CAD build for the part. Positions are in the model's coordinates, mm. A direction names the side the tool comes from. Give positions to 0.01 mm unless a question says otherwise; leave off trailing zeros. Order: outer loops, then holes, each group sorted by start corner. A loop starts at its lowest first (then second) coordinate and runs counter-clockwise, first axis right, second up.
Item 1: Flat gauge pins, fed straight in: P1, Ø13, axis at x = 142, z = 17, coming from the -Y side; P2, Ø1, axis at x = 159, y = -9.5, coming from the -Z side; P3, Ø7.5, axis at y = -12, z = 16.5, coming from the +X side. Where does each tip first touch, or does it go through?
Item 2: Band-saw the part on B-B on y = 0. Give the cut face in (x, z).
Item 3: Band-saw the part on D-D on x = 172. Give the cut face in (y, z), plus the area to 3 significant figures.
Item 4: Band-saw the part on A-A on x = 97.5. Give the cut face in (y, z).
Item 5: Wall check: L1, parallel to X at y = -23.5, z = 25; L2, parallel to X at y = -13, z = 36; L3, parallel to X at y = 27, z = 25. Give the ranges that are in metal, low to high.
Item 6: Band-saw the part on C-C on z = 15.5. Count the separate pieces of the cut face and the enclosed holes in it, plus the area to 3 significant figures.
Item 7: Which spindle directions (+Z, -Z, +X, -X, +Y, -Y) get a long thin tool onto all of the face, cutting with end or side? Do faces 5 (the flat face through (206, -40.5, 11)), 6 (the flat face through (3, -25, 10)), 7 (the flat face through (7.08, 34, 4)). Say none if no direction does.
Item 8: Two-plate mould, pull along Y, no slides. Class faces 1 (the cylindrical face through (102.59, 1.01, 45.71)), 2 (the flat face through (9, 0, 23.64)), 3 (the cylindrical face through (9.136, 38.751, 12.245)), 4 (the flat face through (206, -1, 26.25)): released by +Y, released by -Y, zero draft, split by the parting line, or undercut.
```python
from build123d import *

# Parameters (mm, degrees)
REVOLVE2_ANGLE           = 180
SKETCH5_W                = 2.54
SKETCH5_H                = 12.7
SKETCH5_W_2              = 101.6
SKETCH5_H_2              = 2.54
SKETCH5_W_3              = 12.7
BOSS_EXTRUDE1_DEPTH      = 2.54
SKETCH7_W                = 20
SKETCH7_H                = 50
CUT_EXTRUDE1_DEPTH       = 7
BOSS_EXTRUDE3_REACH      = 220.035
SKETCH8_W                = 5
SKETCH8_H                = 91.44
SKETCH9_W                = 6.129296028
SKETCH9_H                = 8.078685473
BOSS_EXTRUDE4_DEPTH      = 2
BOSS_EXTRUDE7_START      = 8
BOSS_EXTRUDE7_DEPTH      = 8
BOSS_EXTRUDE8_REACH      = 220.035
BOSS_EXTRUDE8_END_RADIUS = 40.64
SKETCH13_W               = 75.08
SKETCH13_H               = 60.08
SKETCH13_W_2             = 70
SKETCH13_H_2             = 55
SKETCH14_W               = 75.08
SKETCH14_H               = 60.08
CUT_EXTRUDE3_DEPTH       = 11
BOSS_EXTRUDE9_REACH      = 217.997
SKETCH15_W               = 70
SKETCH15_H               = 55
CUT_EXTRUDE5_DEPTH       = 15
CUT_EXTRUDE6_REACH       = 202.84
SKETCH18_W               = 12
SKETCH18_H               = 56
BOSS_EXTRUDE10_REACH     = 220.035
SKETCH23_W               = 10
SKETCH23_H               = 81.28
SKETCH24_W               = 26.25
SKETCH24_H               = 81
CUT_EXTRUDE7_DEPTH       = 5.25


with BuildPart() as part:
    # Sketch2 → Revolve2 (revolve)
    with BuildSketch(Plane.XY):
        Polygon((0, 0), (0, 40.64), (0, 45.72), (25.4, 45.72), (195.4, 45.72), (208.1, 45.72), (208.22771659, 40.64), (195.52771659, 40.64), (25.4, 40.64), (5.08, 40.64), (5.08, 0), align=None)
    revolve(axis=Axis((0, 0, 0), (1, 0, 0)), revolution_arc=REVOLVE2_ANGLE)

    # Sketch5 → Boss-Extrude1 (add)
    with BuildSketch(Plane(origin=(0, 0, 0), x_dir=(-1, 0, 0), z_dir=(0, 0, -1))):
        with Locations((-2.54, 34.29)):
            Rectangle(SKETCH5_W, SKETCH5_H)
        with Locations((-104.113858295, -43.18)):
            Rectangle(SKETCH5_W_2, SKETCH5_H_2)
        with Locations((-11.43, 43.18)):
            Rectangle(SKETCH5_W_3, SKETCH5_H_2)
        with Locations((-104.113858295, 43.18)):
            Rectangle(SKETCH5_W_2, SKETCH5_H_2)
        with Locations((-11.43, -43.18)):
            Rectangle(SKETCH5_W_3, SKETCH5_H_2)
        with Locations((-2.54, -34.29)):
            Rectangle(SKETCH5_W, SKETCH5_H)
    extrude(amount=BOSS_EXTRUDE1_DEPTH)

    # Sketch7 → Cut-Extrude1 (cut)
    with BuildSketch(Plane.ZY):
        with Locations((10, 0)):
            Rectangle(SKETCH7_W, SKETCH7_H)
    extrude(amount=-CUT_EXTRUDE1_DEPTH, mode=Mode.SUBTRACT)

    # Sketch8 → Boss-Extrude3 (add, up to next)
    with BuildSketch(Plane(origin=(0, 0, 0), x_dir=(-1, 0, 0), z_dir=(0, 0, -1)), mode=Mode.PRIVATE) as boss_extrude3_sk1:
        with Locations((-15.58, 0)):
            Rectangle(SKETCH8_W, SKETCH8_H)
    boss_extrude3_tool1 = extrude(boss_extrude3_sk1.sketch, amount=-BOSS_EXTRUDE3_REACH, mode=Mode.PRIVATE) - part.part
    add(boss_extrude3_tool1.solids().sort_by_distance((15.58, 0, 0))[0])

    # Sketch9 → Boss-Extrude4 (add)
    with BuildSketch(Plane(origin=(5.08, 0, 0), x_dir=(0, 0, -1), z_dir=(1, 0, 0))):
        with Locations((-3.906446672, 33.952493663)):
            Rectangle(SKETCH9_W, SKETCH9_H)
    extrude(amount=BOSS_EXTRUDE4_DEPTH)

    # Sketch12 → Boss-Extrude7 (add)
    with BuildSketch(Plane.ZY.offset(-13.08).offset(BOSS_EXTRUDE7_START)):
        with BuildLine():
            Line((23.64, 33.056920607), (23.64, -33.056920607))
            ThreePointArc((23.64, -33.056920607), (40.64, 0), (23.64, 33.056920607))
        make_face()
    extrude(amount=-BOSS_EXTRUDE7_DEPTH)

    # Boss-Extrude8: up to this cylinder (the profile starts inside it)
    boss_extrude8_end = Plane(origin=(148.153858, 0, 0), z_dir=(-1, 0, 0)) * Cylinder(BOSS_EXTRUDE8_END_RADIUS, 522.35, mode=Mode.PRIVATE)
    # Sketch13 → Boss-Extrude8 (add, up to the surface)
    with BuildSketch(Plane(origin=(0, 0, 0), x_dir=(-1, 0, 0), z_dir=(0, 0, -1)), mode=Mode.PRIVATE) as boss_extrude8_sk1:
        with Locations((-148.153858295, 0)):
            Rectangle(SKETCH13_W, SKETCH13_H)
        with Locations((-148.153858295, 0)):
            Rectangle(SKETCH13_W_2, SKETCH13_H_2, mode=Mode.SUBTRACT)
    boss_extrude8_tool1 = extrude(boss_extrude8_sk1.sketch, amount=-BOSS_EXTRUDE8_REACH, mode=Mode.PRIVATE) & boss_extrude8_end
    add(boss_extrude8_tool1.solids().sort_by_distance((148.153858, 29.078407, 0))[0])

    # Sketch14 → Cut-Extrude3 (cut)
    with BuildSketch(Plane(origin=(0, 0, 0), x_dir=(-1, 0, 0), z_dir=(0, 0, -1))):
        with Locations((-148.153858295, 0)):
            Rectangle(SKETCH14_W, SKETCH14_H)
    extrude(amount=-CUT_EXTRUDE3_DEPTH, mode=Mode.SUBTRACT)

    # Sketch15 → Boss-Extrude9 (add, up to next)
    with BuildSketch(Plane(origin=(0, 0, 11), x_dir=(-1, 0, 0), z_dir=(0, 0, -1)), mode=Mode.PRIVATE) as boss_extrude9_sk1:
        with Locations((-148.153858295, 0)):
            Rectangle(SKETCH15_W, SKETCH15_H)
    boss_extrude9_tool1 = extrude(boss_extrude9_sk1.sketch, amount=-BOSS_EXTRUDE9_REACH, mode=Mode.PRIVATE) - part.part
    add(boss_extrude9_tool1.solids().sort_by_distance((148.153858, 0, 11))[0])

    # Sketch17 → Cut-Extrude5 (cut)
    with BuildSketch(Plane(origin=(0, 0, 11), x_dir=(-1, 0, 0), z_dir=(0, 0, -1))):
        Polygon((-113.153858295, 27.5), (-183.153858295, 27.5), (-183.153858295, 19.5), (-185.693858295, 19.5), (-185.693858295, 5.5), (-183.153858295, 5.5), (-183.153858295, -13.5), (-185.693858295, -13.5), (-185.693858295, -24.5), (-183.153858295, -24.5), (-183.153858295, -27.5), (-113.153858295, -27.5), align=None)
    extrude(amount=-CUT_EXTRUDE5_DEPTH, mode=Mode.SUBTRACT)

    # Sketch18 → Cut-Extrude6 (cut, up to next)
    with BuildSketch(Plane(origin=(18.08, 0, 0), x_dir=(0, 0, -1), z_dir=(1, 0, 0)), mode=Mode.PRIVATE) as cut_extrude6_sk1:
        with Locations((-6, -10.004795356)):
            Rectangle(SKETCH18_W, SKETCH18_H)
    cut_extrude6_tool1 = extrude(cut_extrude6_sk1.sketch, amount=-CUT_EXTRUDE6_REACH, mode=Mode.PRIVATE) & part.part
    add(cut_extrude6_tool1.solids().sort_by_distance((18.08, -10.004795, 6))[0], mode=Mode.SUBTRACT)

    # Sketch23 → Boss-Extrude10 (add, up to next)
    with BuildSketch(Plane(origin=(0, 0, 0), x_dir=(-1, 0, 0), z_dir=(0, 0, -1)), mode=Mode.PRIVATE) as boss_extrude10_sk1:
        with Locations((-203.22771659, 0)):
            Rectangle(SKETCH23_W, SKETCH23_H)
    boss_extrude10_tool1 = extrude(boss_extrude10_sk1.sketch, amount=-BOSS_EXTRUDE10_REACH, mode=Mode.PRIVATE) - part.part
    add(boss_extrude10_tool1.solids().sort_by_distance((203.227717, 0, 0))[0])

    # Sketch24 → Cut-Extrude7 (cut)
    with BuildSketch(Plane(origin=(208.22771659, 0, 0), x_dir=(0, 0, -1), z_dir=(1, 0, 0))):
        with Locations((-13.125, 0)):
            Rectangle(SKETCH24_W, SKETCH24_H)
    extrude(amount=-CUT_EXTRUDE7_DEPTH, mode=Mode.SUBTRACT)


solid = part.part
```
The answers:
1. P1: stops at y = -44.5
1. P2: stops at z = 26
1. P3: stops at x = 202.98
2. outline: (0, 20) - (5.08, 20) - (5.08, 23.64) - (13.08, 23.64) - (13.08, 12) - (18.08, 12) - (18.08, 40.64) - (110.61, 40.64) - (110.61, 11) - (113.15, 11) - (113.15, 26) - (183.15, 26) - (183.15, 11) - (185.69, 11) - (185.69, 40.64) - (198.23, 40.64) - (198.23, 0) - (202.98, 0) - (202.98, 26.25) - (208.23, 26.25) - (208.23, 40.64) - (208.1, 45.72) - (0, 45.72) - close
3. outline: (-45.72, 0) - (-40.64, 0) arc R40.64 cw to (-30.04, 27.37) - (-30.04, 11) - (-27.5, 11) - (-27.5, 26) - (27.5, 26) - (27.5, 11) - (30.04, 11) - (30.04, 27.37) arc R40.64 cw to (40.64, 0) - (45.72, 0) arc R45.72 ccw to start
3. area: 1,400 mm2
4. outline: (-45.72, 0) - (-44.45, 0) - (-44.45, -2.54) - (-41.91, -2.54) - (-41.91, 0) - (-40.64, 0) arc R40.64 cw to (40.64, 0) - (41.91, 0) - (41.91, -2.54) - (44.45, -2.54) - (44.45, 0) - (45.72, 0) arc R45.72 ccw to start
5. L1: x = 0 to 18.08, 110.61 to 113.15, 198.23 to 202.98
5. L2: x = 0 to 18.08, 110.61 to 185.69, 198.23 to 208.23
5. L3: x = 0 to 18.08, 110.61 to 113.15, 183.15 to 185.69, 198.23 to 202.98
6. separate pieces: 3
6. enclosed holes: 1
6. area: 3,690 mm2
7. face 5: +Z, -Z, +X
7. face 6: -Z, -X
7. face 7: -Z
8. face 1: split by the parting line
8. face 2: undercut
8. face 3: undercut
8. face 4: zero draft
